Geometry check sheet. Reference: drawing and pictorial views, mm from the part's lowest x, y, z. Coordinates: 2 decimals unless noted, no trailing zeros. Loops run counter-clockwise (first coordinate to the right, second up) from the corner with the lowest first, then second, coordinate; pieces in that order, holes last. Notation, with made-up numbers: (-11.75, -11) -> (30.25, -11) arc R6 ccw to (30.25, 0) -> close; hole circle Ø8 at (6.25, -35.75). An arc over 180 degrees is marked (long way). Answer as a JSON object with one key per item and string values. Group by question number.
Q1. Scan lines: L1, parallel to Y at x = 5, z = 1.8; L2, parallel to X at y = 5.5, z = 4.7; L3, parallel to X at y = 6.75, z = 4.7. Record each from-to range of solid material in increasing order.
Q2. Gauge pin test, flat end, axial feed: pin 1 Ø6 at (x, y) = (5, 5) entering from -Z. Record the tip position at first contact, or that the pin passes through.
Q3. Cross-section at C-C on z = 2.4. Record the boundary of the cut face in (x, y), and give its area (3 significant figures).
Q4. Cross-section at B-B on y = 5. Record the boundary of the cut face in (x, z), and give its area (4 significant figures).
Q5. Cross-section at A-A on x = 5. Record the boundary of the cut face in (y, z), and give its area (3 significant figures).
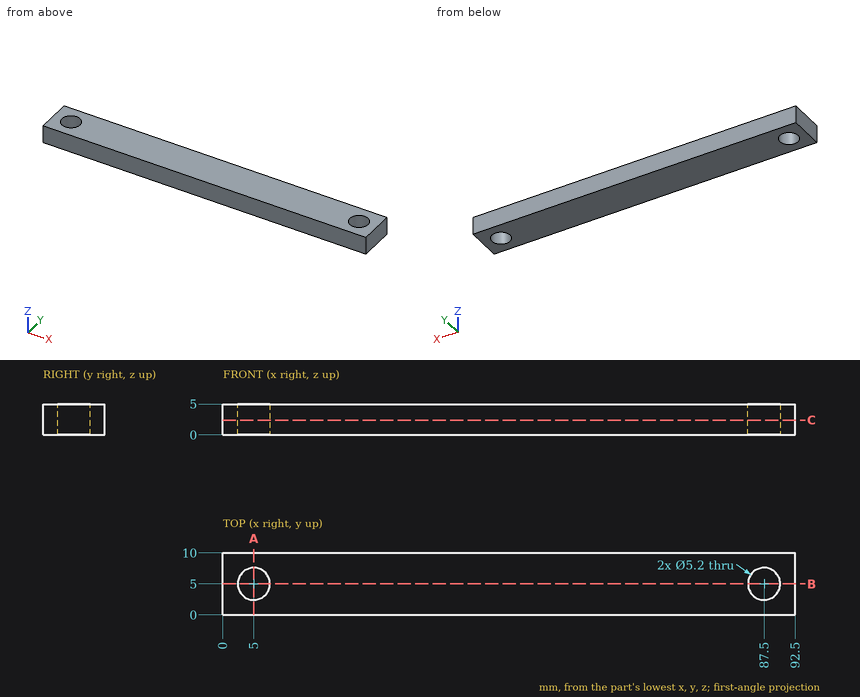
Computed values:
{
 "1": {"L1": "y = 0 to 2.4, 7.6 to 10", "L2": "x = 0 to 2.45, 7.55 to 84.95, 90.05 to 92.5", "L3": "x = 0 to 3.08, 6.92 to 85.58, 89.42 to 92.5"},
 "2": {"pin 1": "stops at z = 0"},
 "3": {"outline": "(0, 0) -> (92.5, 0) -> (92.5, 10) -> (0, 10) -> close; hole circle Ø5.2 at (5, 5); hole circle Ø5.2 at (87.5, 5)", "area": "883 mm²"},
 "4": {"outline": "(0, 0) -> (2.4, 0) -> (2.4, 5) -> (0, 5) -> close; (7.6, 0) -> (84.9, 0) -> (84.9, 5) -> (7.6, 5) -> close; (90.1, 0) -> (92.5, 0) -> (92.5, 5) -> (90.1, 5) -> close", "area": "410.5 mm²"},
 "5": {"outline": "(0, 0) -> (2.4, 0) -> (2.4, 5) -> (0, 5) -> close; (7.6, 0) -> (10, 0) -> (10, 5) -> (7.6, 5) -> close", "area": "24.0 mm²"}
}
